Design review of the part built by this model. Coordinates are the model's own, in mm. Face numbers are marked on the shaded views. A direction names the side the tool comes from. Coordinates: 2 decimals unless noted, no trailing zeros. Write each loop counter-clockwise with the first axis right and the second up, starting at its lowest first coordinate (ties: lowest second). Pieces come first, ordered by that corner, then holes. Notation, with made-up numbers: (5, 75.25) -> (26, 75.25) arc R20 cw to (26, 99.25) -> close; hole circle Ø6 at (-19.75, -20). An arc over 180 degrees is marked (long way). Answer in a Markdown table with one row per item. Add a question column.
Item 1: Take a section at C-C, the plane z = 17.5. Write out the cut boundary in (x, y) (3 decimals).
Item 2: Take a section at B-B, the plane z = -13. Write out the cut boundary in (x, y) (3 decimals), and give its area (3 significant figures).
Item 3: To check wall thickness, follow line 1 (X direction, y = 3, z = 13); line 2 (Y direction, x = 1.5, z = 17); line 3 (X direction, y = 7.5, z = 13) (3 decimals). State the ranges of each line that lie inside material, in increasing order.
Item 4: Take a section at A-A, the plane x = 24.75. Write out the cut boundary in (y, z).
Item 5: Clearance check with flat-ended pins moving along their axes: P1, Ø2.5, axis at x = 24.75, z = 13, coming from the -Y side; P2, Ø1.2, axis at x = 1, y = 8.5, coming from the +Z side; P3, Ø3, axis at x = -22.5, z = -10.5, coming from the +Y side; P4, Ø3.5, axis at y = 8.5, z = 1.5, coming from the +X side (3 decimals). State where each tip first meets the part, or that it passes through.
Item 6: Take a section at D-D, the plane z = -3. Write out the cut boundary in (x, y) (3 decimals), and give its area (3 significant figures).
Item 7: For the marked faces 1, 2 and 3, list the 3-axis set-ups (+Z, -Z, +X, -X, +Y, -Y) from which the entire face can be reached by the end or side of a thin tool; tool diameter is ignored.
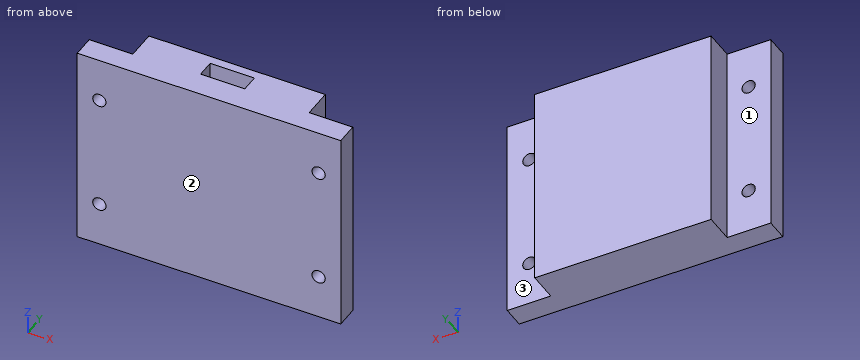
from build123d import *

# Parameters (mm, degrees)
SKETCH_1_W          = 59.5
SKETCH_1_H          = 46
SKETCH_1_R          = 1.5
EXTRUDE_1_DEPTH     = 5
SKETCH_2_W          = 39.81
SKETCH_2_H          = 46
EXTRUDE_2_DEPTH     = 6.7
SKETCH_3_W          = 10
SKETCH_3_H          = 4
CUT_EXTRUDE_1_DEPTH = 6.7


with BuildPart() as part:
    # 草图1 → 凸台-拉伸1 (new body)
    with BuildSketch(Plane(origin=(0, 0, 0), x_dir=(1, 0, 0), z_dir=(0, 1, 0))):
        Rectangle(SKETCH_1_W, SKETCH_1_H)
        with Locations(Location((24.75, 13, 0), (0, 0, 270))):
            Circle(SKETCH_1_R, mode=Mode.SUBTRACT)
        with Locations(Location((24.75, -13, 0), (0, 0, 90))):
            Circle(SKETCH_1_R, mode=Mode.SUBTRACT)
        with Locations(Location((-24.75, -13, 0), (0, 0, 270))):
            Circle(SKETCH_1_R, mode=Mode.SUBTRACT)
        with Locations(Location((-24.75, 13, 0), (0, 0, 90))):
            Circle(SKETCH_1_R, mode=Mode.SUBTRACT)
    extrude(amount=EXTRUDE_1_DEPTH)

    # 草图2 → 凸台-拉伸2 (add)
    with BuildSketch(Plane(origin=(0, 5, 0), x_dir=(1, 0, 0), z_dir=(0, 1, 0))):
        Rectangle(SKETCH_2_W, SKETCH_2_H)
    extrude(amount=EXTRUDE_2_DEPTH)

    # 草图3 → 切除-拉伸1 (cut)
    with BuildSketch(Plane.XY.offset(23)):
        with Locations((0, 7.7)):
            Rectangle(SKETCH_3_W, SKETCH_3_H)
    extrude(amount=-CUT_EXTRUDE_1_DEPTH, mode=Mode.SUBTRACT)


solid = part.part
Answers:
| question | item | result |
|---|---|---|
| 1 | outline | (-29.75, 0) -> (29.75, 0) -> (29.75, 5) -> (19.905, 5) -> (19.905, 11.7) -> (-19.905, 11.7) -> (-19.905, 5) -> (-29.75, 5) -> close; hole (-5, 5.7) -> (5, 5.7) -> (5, 9.7) -> (-5, 9.7) -> close |
| 2 | outline | (-29.75, 0) -> (-26.25, 0) -> (-26.25, 5) -> (-29.75, 5) -> close; (-23.25, 0) -> (23.25, 0) -> (23.25, 5) -> (19.905, 5) -> (19.905, 11.7) -> (-19.905, 11.7) -> (-19.905, 5) -> (-23.25, 5) -> close; (26.25, 0) -> (29.75, 0) -> (29.75, 5) -> (26.25, 5) -> close |
| 2 | area | 534 mm^2 |
| 3 | line 1 | x = -29.75 to -26.25, -23.25 to 23.25, 26.25 to 29.75 |
| 3 | line 2 | y = 0 to 5.7, 9.7 to 11.7 |
| 3 | line 3 | x = -19.905 to 19.905 |
| 4 | outline | (0, -23) -> (5, -23) -> (5, -14.5) -> (0, -14.5) -> close; (0, -11.5) -> (5, -11.5) -> (5, 11.5) -> (0, 11.5) -> close; (0, 14.5) -> (5, 14.5) -> (5, 23) -> (0, 23) -> close |
| 5 | P1 | passes through |
| 5 | P2 | stops at z = 16.3 |
| 5 | P3 | stops at y = 5 |
| 5 | P4 | stops at x = 19.905 |
| 6 | outline | (-29.75, 0) -> (29.75, 0) -> (29.75, 5) -> (19.905, 5) -> (19.905, 11.7) -> (-19.905, 11.7) -> (-19.905, 5) -> (-29.75, 5) -> close |
| 6 | area | 564 mm^2 |
| 7 | face 1 | +Z, -Z, -X, +Y |
| 7 | face 2 | +Z, -Z, +X, -X, -Y |
| 7 | face 3 | +Z, -Z, +X, +Y |
